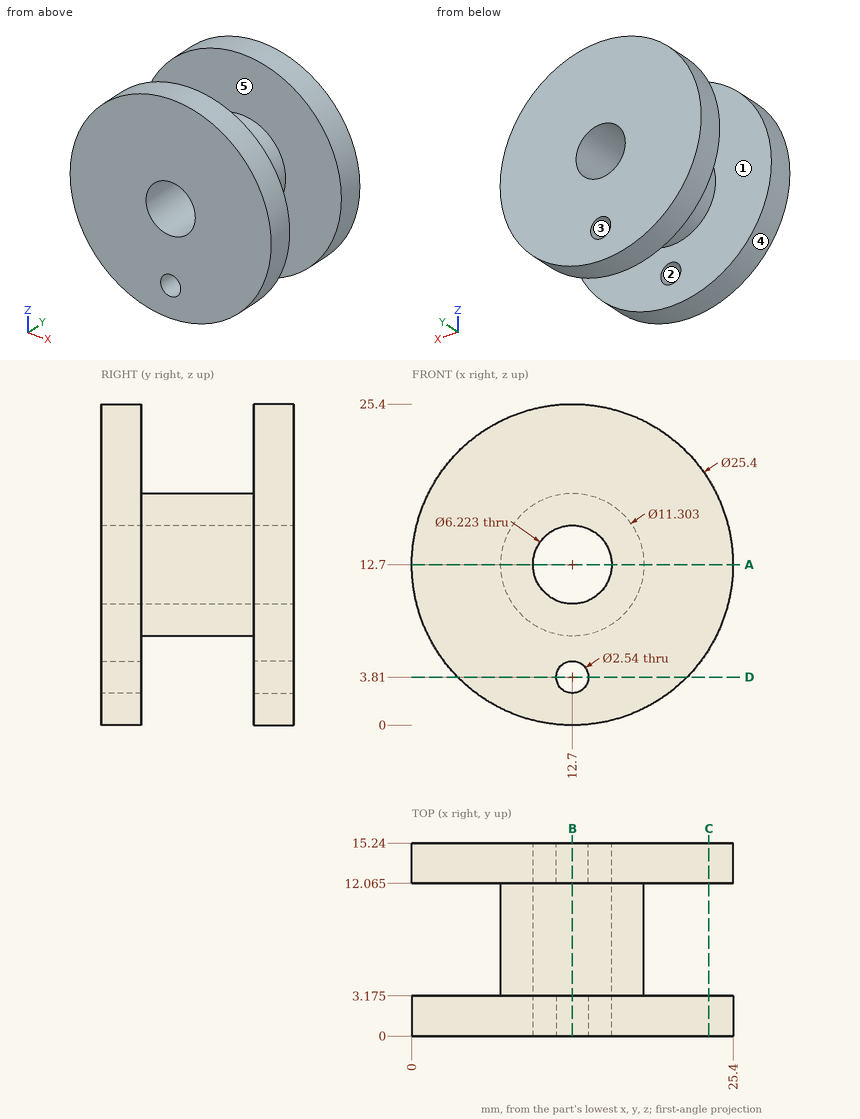
Can you work these out from the drawing? Everything is in mm from the part's minimum corner. A direction names the side the tool comes from. Give positions to 0.01 mm unless a question says otherwise; leave off trailing zeros. Loops run counter-clockwise (first coordinate to the right, second up) from the corner with the lowest first, then second, coordinate; pieces in that order, holes last. Notation, with made-up numbers: (-18.5, 32) -> (29.5, 32) arc R29 cw to (29.5, 61) -> close; hole circle Ø8 at (21.25, -35). An arc over 180 degrees is marked (long way). Write item = value, one per line.
1) For the marked faces 1 and 2, which set-ups out of +Z, -Z, +X, -X, +Y, -Y let a thin tool reach every point of the face, with its end or its side?
Check result:
face_1 = none
face_2 = +Y, -Y
2) Will these pins go through, and if not, where does the flat tip stop? pin 1 (6 mm diameter, centred on y = 3.5, z = 3.5, fed in from -X); pin 2 (1.5 mm diameter, centred on y = 9.5, z = 14, fed in from -X); pin 3 (2 mm diameter, centred on y = 7.5, z = 18.5, fed in from -X).
Check result:
pin_1 = 1.63
pin_2 = 7.08
pin_3 = 9.72
3) Suppose I cut it at B-B on x = 12.7. Write out the boundary of the cut face in (y, z) (1 decimal).
Check result:
outline = (0, 0) -> (3.2, 0) -> (3.2, 2.5) -> (0, 2.5) -> close; (0, 5.1) -> (3.2, 5.1) -> (3.2, 7) -> (12.1, 7) -> (12.1, 5.1) -> (15.2, 5.1) -> (15.2, 9.6) -> (0, 9.6) -> close; (0, 15.8) -> (15.2, 15.8) -> (15.2, 25.4) -> (12.1, 25.4) -> (12.1, 18.4) -> (3.2, 18.4) -> (3.2, 25.4) -> (0, 25.4) -> close; (12.1, 0) -> (15.2, 0) -> (15.2, 2.5) -> (12.1, 2.5) -> close
4) Suppose I cut it at A-A on z = 12.7. Write out the boundary of the cut face in (x, y) (1 decimal), then the cut area to 3 significant figures.
Check result:
outline = (0, 0) -> (9.6, 0) -> (9.6, 15.2) -> (0, 15.2) -> (0, 12.1) -> (7, 12.1) -> (7, 3.2) -> (0, 3.2) -> close; (15.8, 0) -> (25.4, 0) -> (25.4, 3.2) -> (18.4, 3.2) -> (18.4, 12.1) -> (25.4, 12.1) -> (25.4, 15.2) -> (15.8, 15.2) -> close
area = 167 mm2
5) I need wall thicknesses on L1, parallel to Y at x = 6, z = 13.75 (3 decimals); L2, parallel to X at y = 4, z = 12.7; L3, parallel to X at y = 12.5, z = 3. Which ranges of each line are inside material? Lowest first, please. Write a range as from..to.
Check result:
L1 = 0..3.175, 12.065..15.24
L2 = 7.05..9.59, 15.81..18.35
L3 = 4.5..11.72, 13.68..20.9
6) Thinking about a two-plate mould opening in Z: for the marked faces 3, 4 and 5, which applies, released by +Z, released by -Z, zero draft, split by the parting line, or undercut?
Check result:
face_3 = undercut
face_4 = split by the parting line
face_5 = zero draft
7) Suppose I cut it at D-D on z = 3.81. Write out the boundary of the cut face in (x, y) (3 decimals), then the cut area to 3 significant figures.
Check result:
outline = (3.63, 0) -> (11.43, 0) -> (11.43, 3.175) -> (3.63, 3.175) -> close; (3.63, 12.065) -> (11.43, 12.065) -> (11.43, 15.24) -> (3.63, 15.24) -> close; (13.97, 0) -> (21.77, 0) -> (21.77, 3.175) -> (13.97, 3.175) -> close; (13.97, 12.065) -> (21.77, 12.065) -> (21.77, 15.24) -> (13.97, 15.24) -> close
area = 99.1 mm2
8) Suppose I cut it at C-C on x = 23.5. Write out the boundary of the cut face in (y, z) (3 decimals).
Check result:
outline = (0, 6.018) -> (3.175, 6.018) -> (3.175, 19.382) -> (0, 19.382) -> close; (12.065, 6.018) -> (15.24, 6.018) -> (15.24, 19.382) -> (12.065, 19.382) -> close
